For this review, take the finished solid that the model builds, in its own axes (mm). Face numbers are marked on the shaded views. A direction names the side the tool comes from. Round coordinates to 2 decimals unless told otherwise and drop trailing zeros. Loops run counter-clockwise (first coordinate to the right, second up) from the corner with the lowest first, then second, coordinate; pieces in that order, holes last. Notation, with made-up numbers: M 77,16 L 134,16 A27 cw 134,42 Z; hole C -33.5,-11.75 d1. An arc over 180 degrees is marked long. Write item = value, one per line. Start each with the question number.
```python
from build123d import *

# Parameters (mm, degrees)
SKETCH1_W                                       = 19.05
SKETCH1_H                                       = 57.15
SKETCH1_R                                       = 3.96875
SKETCH1_R_2                                     = 6.35
BOSS_EXTRUDE2_DEPTH                             = 9.525
CBORE_FOR_10_SOCKET_HEAD_CAP_SCREW2_D           = 5.1054
CBORE_FOR_10_SOCKET_HEAD_CAP_SCREW2_DEPTH       = 19.05
CBORE_FOR_10_SOCKET_HEAD_CAP_SCREW2_CBORE_D     = 7.9375
CBORE_FOR_10_SOCKET_HEAD_CAP_SCREW2_CBORE_DEPTH = 4.826
CBORE_FOR_10_SOCKET_HEAD_CAP_SCREW2_TIP         = 1.533816902


with BuildPart() as part:
    # Sketch1 → Boss-Extrude2 (new body)
    with BuildSketch(Plane.XY):
        with Locations((0, -200.025)):
            Rectangle(SKETCH1_W, SKETCH1_H)
        with Locations(Location((0, -200.025, 0), (0, 0, 180))):
            Circle(SKETCH1_R, mode=Mode.SUBTRACT)
        with Locations(Location((0, -180.975, 0), (0, 0, 180))):
            Circle(SKETCH1_R_2, mode=Mode.SUBTRACT)
        with Locations(Location((0, -219.075, 0), (0, 0, 180))):
            Circle(SKETCH1_R_2, mode=Mode.SUBTRACT)
    extrude(amount=BOSS_EXTRUDE2_DEPTH)

    # CBORE for #10 Socket Head Cap Screw2
    with Locations(Plane(origin=(9.525, 0, 0), x_dir=(0, 0, -1), z_dir=(1, 0, 0))):
        with Locations((-4.7625, -200.025)):
            CounterBoreHole(CBORE_FOR_10_SOCKET_HEAD_CAP_SCREW2_D / 2, CBORE_FOR_10_SOCKET_HEAD_CAP_SCREW2_CBORE_D / 2, CBORE_FOR_10_SOCKET_HEAD_CAP_SCREW2_CBORE_DEPTH, depth=CBORE_FOR_10_SOCKET_HEAD_CAP_SCREW2_DEPTH)
            with Locations((0, 0, -(CBORE_FOR_10_SOCKET_HEAD_CAP_SCREW2_DEPTH + CBORE_FOR_10_SOCKET_HEAD_CAP_SCREW2_TIP / 2))):  # 118° drill point
                Cone(0, CBORE_FOR_10_SOCKET_HEAD_CAP_SCREW2_D / 2, CBORE_FOR_10_SOCKET_HEAD_CAP_SCREW2_TIP, mode=Mode.SUBTRACT)


solid = part.part
```
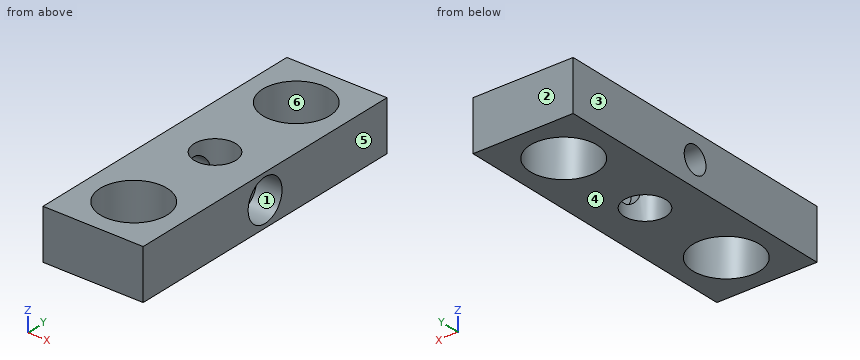
(1) Draft analysis for pull direction X (two halves, no side actions). For the marked faces 3, 4, 5 and 6, state which applies: +X half, -X half, draft (parallel to the pull), parting line (faces both ways), or undercut.
(2) Add section C-C on x = 5.5. Count the separate pieces of the cut face and the enclosed holes in it, and give its area (3 significant figures).
(3) Add section A-A on x = 0. Write out the cut boundary in (y, z) (3 decimals), and give its area (3 significant figures).
(4) Wall thickness on L1, parallel to Y at x = 0, z = 2 (3 decimals); L2, parallel to Y at x = 0.75, z = 7.25; L3, parallel to Y at x = 5.5, z = 0.5: over which ranges is each line inside the solid? List them lowest first.
(5) Add section B-B on y = -216. Write out the cut boundary in (x, z) (3 decimals).
(6) Tool access review of the marked faces 1 and 2: name each direction out of +Z, -Z, +X, -X, +Y, -Y from which nothing blocks a thin tool from reaching the whole face with its end or side.
Answer sheet:
q1.face_3 = -X half
q1.face_4 = draft
q1.face_5 = +X half
q1.face_6 = undercut
q2.separate_pieces = 3
q2.enclosed_holes = 1
q2.area = 374 mm²
q3.outline = M -228.6,0 L -225.425,0 L -225.425,9.525 L -228.6,9.525 Z; M -212.725,0 L -203.994,0 L -203.994,9.525 L -212.725,9.525 Z; M -196.056,0 L -187.325,0 L -187.325,9.525 L -196.056,9.525 Z; M -174.625,0 L -171.45,0 L -171.45,9.525 L -174.625,9.525 Z
q3.area = 227 mm²
q4.L1 = -228.6 to -225.425, -212.725 to -203.994, -196.056 to -187.325, -174.625 to -171.45
q4.L2 = -228.6 to -225.38, -212.77 to -203.92, -196.13 to -187.28, -174.67 to -171.45
q4.L3 = -228.6 to -222.25, -215.9 to -184.15, -177.8 to -171.45
q5.outline = M -9.525,0 L -5.556,0 L -5.556,9.525 L -9.525,9.525 Z; M 5.556,0 L 9.525,0 L 9.525,9.525 L 5.556,9.525 Z
q6.face_1 = +X
q6.face_2 = +Z, -Z, +X, -X, +Y
